Design review of the part shown in the three views and the two pictorial views. Dimensions are in mm from the part's minimum x, y and z. A direction names the side the tool comes from. Round coordinates to 2 decimals unless told otherwise and drop trailing zeros. Loops run counter-clockwise (first coordinate to the right, second up) from the corner with the lowest first, then second, coordinate; pieces in that order, holes last. Notation, with made-up numbers: (-37.75, 87) -> (-21.75, 87) arc R22 ccw to (-21.75, 105) -> close; hole circle Ø10 at (-0.75, -13). An arc over 180 degrees is marked (long way). Write each question's results on one line, items separated by ' | '. Start each with the question number.
Item 1: For L1, parallel to Y at x = 4, z = 9.25; L2, parallel to Z at x = 5.5, y = 2.75; L3, parallel to X at y = 5, z = 6.5 (1 decimal), list the stretches that pass through material, from the lowest coordinate up. Write a range as from..to.
Item 2: We need section A-A (z = 4.25). Give the boundary of the cut face in (x, y).
Item 3: Tool access review of the marked faces 4 and 5: name each direction out of +Z, -Z, +X, -X, +Y, -Y from which nothing blocks a thin tool from reaching the whole face with its end or side.
Item 4: Clearance check with flat-ended pins moving along their axes: pin 1 Ø3.5 at (x, y) = (4, 4) entering from -Z; pin 2 Ø3 at (y, z) = (7, 1.5) entering from -X; pin 3 Ø1.5 at (x, z) = (2.5, 3.5) entering from -Y. State where each tip first meets the part, or that it passes through.
Item 5: We need section B-B (x = 4). Give the boundary of the cut face in (y, z).
Item 6: Mouldability with a two-part tool opening along Y and no side actions: class the marked faces 1, 2 and 3 as pulls with the +Y half, pulls with the -Y half, needs draft (parallel to the pull), parting line crosses it, or undercut.
Item 7: We need section C-C (z = 9). Give the boundary of the cut face in (x, y).
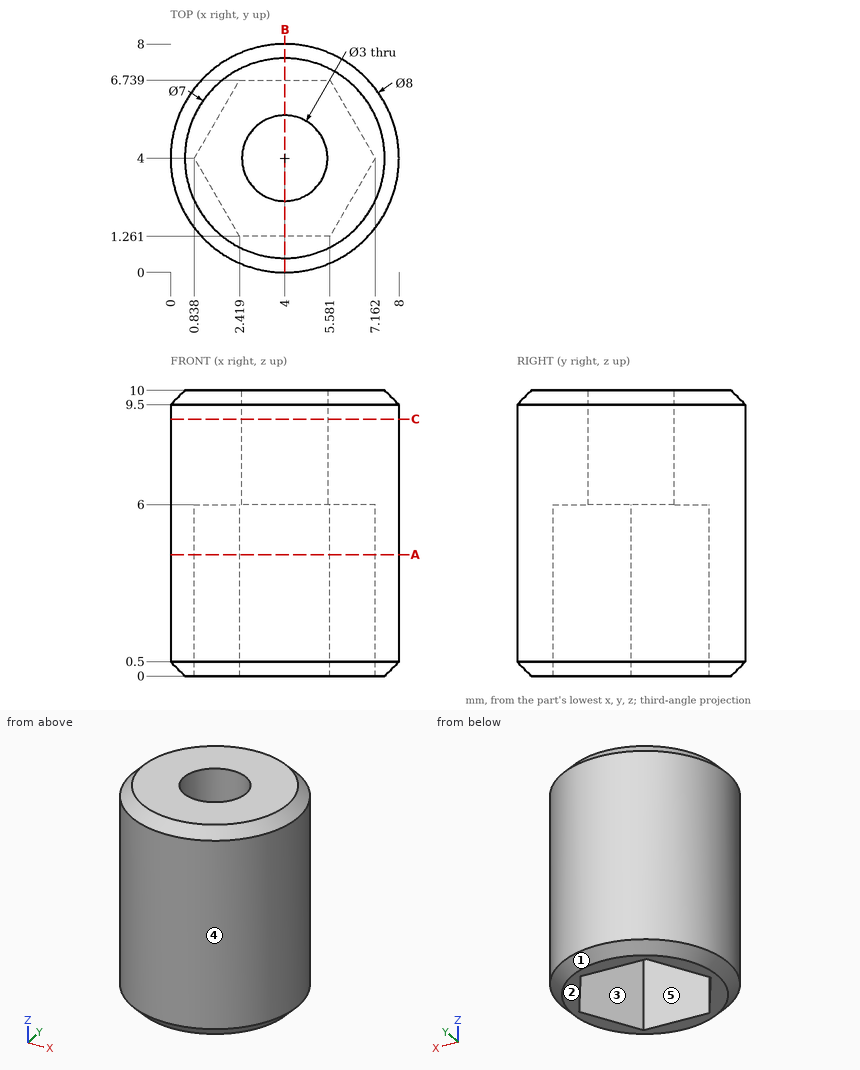
Here are the results:
1) L1: y = 0..2.5, 5.5..8 | L2: z = 6..10 | L3: x = 0.1..2.9, 5.1..7.9
2) outline: circle Ø8 at (4, 4); hole (0.84, 4) -> (2.42, 1.26) -> (5.58, 1.26) -> (7.16, 4) -> (5.58, 6.74) -> (2.42, 6.74) -> close
3) face 4: +Z, -Z | face 5: -Z
4) pin 1: stops at z = 6 | pin 2: stops at x = 0.29 | pin 3: stops at y = 0.07
5) outline: (0, 0.5) -> (0.5, 0) -> (1.26, 0) -> (1.26, 6) -> (2.5, 6) -> (2.5, 10) -> (0.5, 10) -> (0, 9.5) -> close; (5.5, 6) -> (6.74, 6) -> (6.74, 0) -> (7.5, 0) -> (8, 0.5) -> (8, 9.5) -> (7.5, 10) -> (5.5, 10) -> close
6) face 1: parting line crosses it | face 2: needs draft | face 3: undercut
7) outline: circle Ø8 at (4, 4); hole circle Ø3 at (4, 4)
